from build123d import *

# Parameters (mm, degrees)
F0_R     = 2
F1_DEPTH = 3
F2_R     = 0.3
F3_R     = 0.3


with BuildPart() as f1:
    # F0 (on Top) → F1 (new body)
    with BuildSketch(Plane.XY):
        Polygon((3.999987, -0.010358), (2.008964, 3.458911), (-1.991023, 3.469269), (-3.999987, 0.010358), (-2.008964, -3.458911), (1.991023, -3.469269), align=None)
        Circle(F0_R, mode=Mode.SUBTRACT)
    extrude(amount=F1_DEPTH)

    # F2
    f2_edges = [f1.edges().sort_by_distance(p)[0] for p in [
        (3.004475, 1.724276, 3),
        (0.00897, 3.46409, 3),
        (-2.995505, 1.739814, 3),
        (-3.004475, -1.724276, 3),
        (-0.00897, -3.46409, 3),
        (2.995505, -1.739814, 3),
        (-2, 0, 3),
    ]]
    fillet(f2_edges, radius=F2_R)

    # F3
    f3_edges = [f1.edges().sort_by_distance(p)[0] for p in [
        (3.004475, 1.724276, 0),
        (0.00897, 3.46409, 0),
        (-2.995505, 1.739814, 0),
        (-3.004475, -1.724276, 0),
        (-0.00897, -3.46409, 0),
        (2.995505, -1.739814, 0),
        (-2, 0, 0),
    ]]
    fillet(f3_edges, radius=F3_R)


solid = f1.part
Geometry: final body of the model. Coordinates: model frame, mm. Give positions to 0.01 mm unless a question says otherwise; leave off trailing zeros. Order: outer loops, then holes, each group sorted by start corner. A loop starts at its lowest first (then second) coordinate and runs counter-clockwise, first axis right, second up. Notation, with made-up numbers: (28, 48.25) -> (81, 48.25) arc R30 ccw to (81, 82.25) -> close; hole circle Ø9 at (5.5, 67.5). An arc over 180 degrees is marked (long way). Answer as a JSON object with one key per item and string values.
Q1. First-contact query: pin 1 (3 mm diameter, centred on x = 0.5, y = 0.5, fed in from +Z); pin 2 (1.5 mm diameter, centred on x = -1, y = -0.5, fed in from +Z); pin 3 (1 mm diameter, centred on y = 2.5, z = 0.5, fed in from +X). Flat tips, straight axial feed; report the tip coordinate or a pass-through.
Entries:
{"pin 1": "stops at z = 2.99", "pin 2": "passes through", "pin 3": "stops at x = 2.85"}
Q2. Draft query along Y for faces 1 (the flat face through (2.4, 0.7, 3)), 2 (the cylindrical face through (0, -2, 1)), 3 (the cylindrical face through (-2.94, 1.67, 2.91)). Return one class per face: released by +Y, released by -Y, zero draft, split by the parting line, or undercut.
Entries:
{"face 1": "zero draft", "face 2": "undercut", "face 3": "released by +Y"}
Q3. Section B-B (z = 0.2). Output: boundary loops of the cut face in (x, y), plus the area to 3 significant figures.
Entries:
{"outline": "(-3.98, 0.01) -> (-2, -3.44) -> (1.98, -3.45) -> (3.98, -0.01) -> (2, 3.44) -> (-1.98, 3.45) -> close; hole circle Ø4.03 at (0, 0)", "area": "28.4 mm^2"}
Q4. Section A-A (z = 1.05). Output: boundary loops of the cut face in (x, y).
Entries:
{"outline": "(-4, 0.01) -> (-2.01, -3.46) -> (1.99, -3.47) -> (4, -0.01) -> (2.01, 3.46) -> (-1.99, 3.47) -> close; hole circle Ø4 at (0, 0)"}
Q5. Material intervals for probe 1 along Y at (x, z) = (0.5, 2.3); probe 2 along Y at (x, z) = (0, 1.8); probe 3 along X at (y, z) = (-1, 1.7), sorted ascending.
Entries:
{"probe 1": "y = -3.47 to -1.94, 1.94 to 3.46", "probe 2": "y = -3.46 to -2, 2 to 3.46", "probe 3": "x = -3.42 to -1.73, 1.73 to 3.43"}
